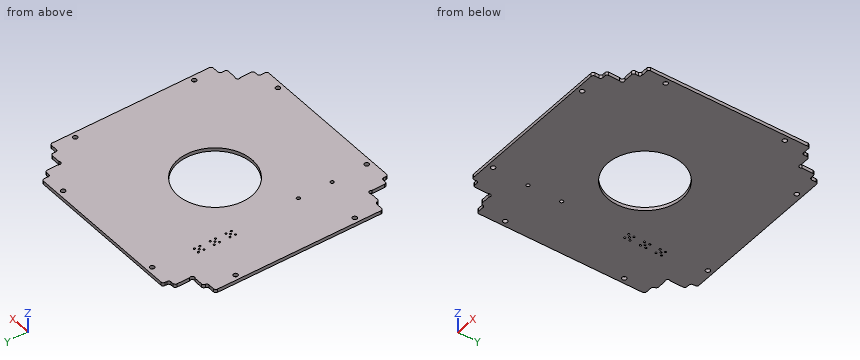
```python
from build123d import *

# Parameters (mm, degrees)
SKETCH1_W            = 106
SKETCH1_H            = 106
MAINOUTLINE_DEPTH    = 1.6
RAILCUTOUTS_DEPTH    = 75.970394157
DOGBONES_DEPTH       = 75.970394157
SOLARFILLETS_DEPTH   = 75.970394157
HANDLINGFILLETS_R    = 1
SKETCH7_R            = 0.8
SKETCH7_R_2          = 0.425
CONNECTORHOLES_DEPTH = 75.9703943
M2_CLEARANCE_HOLE1_D = 2.1
SKETCH10_R           = 17.5
CUT_EXTRUDE1_DEPTH   = 75.9703943


with BuildPart() as part:
    # Sketch1 → mainOutline (new body)
    with BuildSketch(Plane.XY):
        Rectangle(SKETCH1_W, SKETCH1_H)
    extrude(amount=MAINOUTLINE_DEPTH)

    # Sketch4 → railCutouts (cut, through all)
    with BuildSketch(Plane(origin=(0, 0, 0), x_dir=(-1, 0, 0), z_dir=(0, 0, -1))):
        Polygon((-41.4, -41.4), (-48, -41.4), (-48, -39), (-49.9975, -39), (-60.106513243, -39), (-60.106513243, -61.452099286), (-39, -61.452099286), (-39, -49.9), (-39, -49), (-41.4, -49), align=None)
        Polygon((39, -56.27525328), (39, -49.9), (41.4, -49.9), (41.4, -41.4), (48, -41.4), (48, -40.5), (55.517672261, -40.5), (55.517672261, -56.27525328), align=None)
        Polygon((55.383846757, 40.5), (48, 40.5), (48, 41.4), (41.4, 41.4), (41.4, 49.9), (39, 49.9), (39, 57.687687567), (55.383846757, 57.687687567), align=None)
        Polygon((-39, 59.880423019), (-39, 49.9), (-39, 49), (-41.4, 49), (-41.4, 41.4), (-48, 41.4), (-48, 39), (-49.9975, 39), (-56.842822937, 39), (-56.842822937, 59.880423019), align=None)
    extrude(amount=-RAILCUTOUTS_DEPTH, mode=Mode.SUBTRACT)

    # Sketch5 → dogbones (cut, through all)
    with BuildSketch(Plane(origin=(0, 0, 0), x_dir=(-1, 0, 0), z_dir=(0, 0, -1))):
        with BuildLine():
            Line((-41.4, -42.814213562), (-44.73741596, -46.151629522))
            ThreePointArc((-44.73741596, -46.151629522), (-46.151629522, -46.151629522), (-46.151629522, -44.73741596))
            Line((-46.151629522, -44.73741596), (-42.814213562, -41.4))
            ThreePointArc((-42.814213562, -41.4), (-41.4, -41.4), (-41.4, -42.814213562))
        make_face()
        with BuildLine():
            Line((42.814213562, -41.4), (44.747298889, -43.333085326))
            ThreePointArc((44.747298889, -43.333085326), (44.747298889, -44.747298889), (43.333085326, -44.747298889))
            Line((43.333085326, -44.747298889), (41.4, -42.814213562))
            ThreePointArc((41.4, -42.814213562), (41.4, -41.4), (42.814213562, -41.4))
        make_face()
        with BuildLine():
            Line((41.4, 42.814213562), (43.321909081, 44.736122643))
            ThreePointArc((43.321909081, 44.736122643), (44.736122643, 44.736122643), (44.736122643, 43.321909081))
            Line((44.736122643, 43.321909081), (42.814213562, 41.4))
            ThreePointArc((42.814213562, 41.4), (41.4, 41.4), (41.4, 42.814213562))
        make_face()
        with BuildLine():
            Line((-42.814213562, 41.4), (-44.503927418, 43.089713856))
            ThreePointArc((-44.503927418, 43.089713856), (-44.503927418, 44.503927418), (-43.089713856, 44.503927418))
            Line((-43.089713856, 44.503927418), (-41.4, 42.814213562))
            ThreePointArc((-41.4, 42.814213562), (-41.4, 41.4), (-42.814213562, 41.4))
        make_face()
    extrude(amount=-DOGBONES_DEPTH, mode=Mode.SUBTRACT)

    # Sketch6 → solarFillets (cut, through all)
    with BuildSketch(Plane(origin=(0, 0, 0), x_dir=(-1, 0, 0), z_dir=(0, 0, -1))):
        with BuildLine():
            Line((-40, 50), (-40, 53))
            ThreePointArc((-40, 53), (-39, 54), (-38, 53))
            Line((-38, 53), (-38, 50))
            ThreePointArc((-38, 50), (-39, 49), (-40, 50))
        make_face()
        with BuildLine():
            Line((-49, 38), (-53, 38))
            ThreePointArc((-53, 38), (-54, 39), (-53, 40))
            Line((-53, 40), (-49, 40))
            ThreePointArc((-49, 40), (-48, 39), (-49, 38))
        make_face()
        with BuildLine():
            Line((-49, -40), (-55.214202913, -40))
            ThreePointArc((-55.214202913, -40), (-56.214202913, -39), (-55.214202913, -38))
            Line((-55.214202913, -38), (-49, -38))
            ThreePointArc((-49, -38), (-48, -39), (-49, -40))
        make_face()
        with BuildLine():
            Line((-38, -50), (-38, -53.916094318))
            ThreePointArc((-38, -53.916094318), (-39, -54.916094318), (-40, -53.916094318))
            Line((-40, -53.916094318), (-40, -50))
            ThreePointArc((-40, -50), (-39, -49), (-38, -50))
        make_face()
        with BuildLine():
            Line((40, -50.9), (40, -54.538013421))
            ThreePointArc((40, -54.538013421), (39, -55.538013421), (38, -54.538013421))
            Line((38, -54.538013421), (38, -50.9))
            ThreePointArc((38, -50.9), (39, -49.9), (40, -50.9))
        make_face()
        with BuildLine():
            Line((49, -39.5), (54.202622605, -39.5))
            ThreePointArc((54.202622605, -39.5), (55.202622605, -40.5), (54.202622605, -41.5))
            Line((54.202622605, -41.5), (49, -41.5))
            ThreePointArc((49, -41.5), (48, -40.5), (49, -39.5))
        make_face()
        with BuildLine():
            Line((49, 41.5), (54.556563772, 41.5))
            ThreePointArc((54.556563772, 41.5), (55.556563772, 40.5), (54.556563772, 39.5))
            Line((54.556563772, 39.5), (49, 39.5))
            ThreePointArc((49, 39.5), (48, 40.5), (49, 41.5))
        make_face()
        with BuildLine():
            Line((38, 50.9), (38, 55.828092709))
            ThreePointArc((38, 55.828092709), (39, 56.828092709), (40, 55.828092709))
            Line((40, 55.828092709), (40, 50.9))
            ThreePointArc((40, 50.9), (39, 49.9), (38, 50.9))
        make_face()
    extrude(amount=-SOLARFILLETS_DEPTH, mode=Mode.SUBTRACT)

    # handlingFillets
    handlingfillets_edges = [part.edges().sort_by_distance(p)[0] for p in [
        (-41.4, -49.9, 0.8),
        (-38, -53, 0.8),
        (-53, -39.5, 0.8),
        (-48, -41.4, 0.8),
        (-48, 41.4, 0.8),
        (-53, 39.5, 0.8),
        (-41.4, 49.9, 0.8),
        (-38, 53, 0.8),
        (38, 53, 0.8),
        (41.4, 49, 0.8),
        (48, 41.4, 0.8),
        (53, 38, 0.8),
        (53, -38, 0.8),
        (48, -41.4, 0.8),
        (41.4, -49, 0.8),
        (38, -53, 0.8),
    ]]
    fillet(handlingfillets_edges, radius=HANDLINGFILLETS_R)

    # Sketch7 → connectorHoles (cut, through all)
    with BuildSketch(Plane.XY.offset(1.6)):
        with Locations((-28.472296419, -17.925)):
            Circle(SKETCH7_R)
        with Locations((-28.472296419, -33.775)):
            Circle(SKETCH7_R)
        with Locations((-31.37, 28.67)):
            Circle(SKETCH7_R_2)
        with Locations((-28.83, 28.67)):
            Circle(SKETCH7_R_2)
        with Locations((-30.1, 29.94)):
            Circle(SKETCH7_R_2)
        with Locations((-28.83, 31.21)):
            Circle(SKETCH7_R_2)
        with Locations((-31.37, 31.21)):
            Circle(SKETCH7_R_2)
        with Locations((-31.37, 21.27)):
            Circle(SKETCH7_R_2)
        with Locations((-28.83, 21.27)):
            Circle(SKETCH7_R_2)
        with Locations((-30.1, 22.54)):
            Circle(SKETCH7_R_2)
        with Locations((-28.83, 23.81)):
            Circle(SKETCH7_R_2)
        with Locations((-31.37, 23.81)):
            Circle(SKETCH7_R_2)
        with Locations((-31.37, 13.87)):
            Circle(SKETCH7_R_2)
        with Locations((-28.83, 13.87)):
            Circle(SKETCH7_R_2)
        with Locations((-30.1, 15.14)):
            Circle(SKETCH7_R_2)
        with Locations((-28.83, 16.41)):
            Circle(SKETCH7_R_2)
        with Locations((-31.37, 16.41)):
            Circle(SKETCH7_R_2)
    extrude(amount=-CONNECTORHOLES_DEPTH, mode=Mode.SUBTRACT)

    # M2 Clearance Hole1 (through all)
    with Locations(Plane(origin=(0, 0, 0), x_dir=(-1, 0, 0), z_dir=(0, 0, -1))):
        with Locations((50.5, -28), (28, -50.5), (-50.5, -28), (-28, -50.5), (-28, 50.5), (-50.5, 28), (28, 50.5), (50.5, 28)):
            Hole(M2_CLEARANCE_HOLE1_D / 2)

    # Sketch10 → Cut-Extrude1 (cut, through all)
    with BuildSketch(Plane(origin=(0, 0, 0), x_dir=(-1, 0, 0), z_dir=(0, 0, -1))):
        Circle(SKETCH10_R)
    extrude(amount=-CUT_EXTRUDE1_DEPTH, mode=Mode.SUBTRACT)


solid = part.part
```
Verification items for the finished model (mm, model axes). Coordinates: 2 decimals unless noted, no trailing zeros. Loops run counter-clockwise (first coordinate to the right, second up) from the corner with the lowest first, then second, coordinate; pieces in that order, holes last. Notation, with made-up numbers: (51.5, 21) -> (90.5, 21) arc R7 cw to (90.5, 29) -> close; hole circle Ø7 at (42.25, 40.25). An arc over 180 degrees is marked (long way). Answer in a Markdown table with one row per item. Add a question column.
1. Depth check by flat-ended pin: P1, Ø0.8, axis at x = 44, z = 1, coming from the +Y side; P2, Ø0.8, axis at y = 46.5, z = 0.5, coming from the +X side; P3, Ø0.7, axis at x = -40, z = 0.5, coming from the -Y side. Enter the tip coordinate at first touch or a pass-through.
2. Section check A-A, the plane y = 0. Enter the section's corners in (x, z), then the cut area to 3 significant figures.
3. Section check C-C, the plane z = 0.4. Give the number of separate pieces and of enclosed holes in the cut face, then the cut area to 3 significant figures.
4. Material ranges on probe 1 along Y at (x, z) = (50.5, 1); probe 2 along Y at (x, z) = (-27.5, 0.9); probe 3 along X at (y, z) = (-45, 0.55), recorded low to high. Write a range as [from, to].
5. Section check B-B, the plane x = -12.5. Enter the section's corners in (y, z).
Derived:
| question | item | result |
|---|---|---|
| 1 | P1 | stops at y = 41.4 |
| 1 | P2 | stops at x = 41.4 |
| 1 | P3 | stops at y = -49.9 |
| 2 | outline | (-53, 0) -> (-17.5, 0) -> (-17.5, 1.6) -> (-53, 1.6) -> close; (17.5, 0) -> (53, 0) -> (53, 1.6) -> (17.5, 1.6) -> close |
| 2 | area | 114 mm² |
| 3 | separate pieces | 1 |
| 3 | enclosed holes | 26 |
| 3 | area | 9,590 mm² |
| 4 | probe 1 | y = [-38, -29.05], [-26.95, 26.95], [29.05, 38] |
| 4 | probe 2 | y = [-53, -51.42], [-49.58, 49.58], [51.42, 53] |
| 4 | probe 3 | x = [-41.4, 41.4] |
| 5 | outline | (-53, 0) -> (-12.25, 0) -> (-12.25, 1.6) -> (-53, 1.6) -> close; (12.25, 0) -> (53, 0) -> (53, 1.6) -> (12.25, 1.6) -> close |
